CAD build for the part. Positions are in the model's coordinates, mm. A direction names the side the tool comes from. Give positions to 0.01 mm unless a question says otherwise; leave off trailing zeros. Write each loop counter-clockwise with the first axis right and the second up, starting at its lowest first coordinate (ties: lowest second). Pieces come first, ordered by that corner, then holes. Notation, with made-up numbers: (18, 62.5) - (27, 62.5) arc R15 ccw to (27, 73.5) - close; hole circle Ø2 at (75, 84). An arc over 180 degrees is marked (long way). Write item = value, one per line. Start each with the question number.
Autodesk Inventor part; units mm, degrees
ref_plane "YZ Plane" through (0, 0, 0) normal (1, 0, 0) x (0, 1, 0)
ref_plane "XZ Plane" through (0, 0, 0) normal (0, 1, 0) x (-1, 0, 0)
ref_plane "XY Plane" through (0, 0, 0) normal (0, 0, 1) x (1, 0, 0)
sketch "Sketch9" plane through (0, 0, 0) normal (0, 1, 0) x (-1, 0, 0)
  circle A0 centre (0, 0) radius 32
  circle A1 centre (0, 0) radius 47
  circle A2 centre (0, 0) radius 26.5
  dimension "d54" = 64
  dimension "d55" = 94
  dimension "d56" = 53
extrude "Extrusion8" add sketch "Sketch9" against normal blind 4 contours A0
extrude "Extrusion9" add sketch "Sketch9" against normal blind 10 contours A1
sketch "Sketch10" plane through (0, 0, 0) normal (0, 1, 0) x (1, 0, 0)
  circle A0 centre (0, 0) radius 40
  point P0 (-40, 0)
  point P1 (-30.6418, -25.7115)
  point P2 (-6.9459, -39.3923)
  point P3 (20, -34.641)
  point P4 (37.5877, -13.6808)
  point P5 (37.5877, 13.6808)
  point P6 (20, 34.641)
  point P7 (-6.9459, 39.3923)
  point P8 (-30.6418, 25.7115)
  dimension "d61" = 80
  dimension "d64" = 360
hole "Hole1" at (-40, 0, 0) at (-30.6418, 0, 25.7115) at (-6.9459, 0, 39.3923) at (20, 0, 34.641) at (37.5877, 0, 13.6808) at (37.5877, 0, -13.6808) at (20, 0, -34.641) at (-6.9459, 0, -39.3923) at (-30.6418, 0, -25.7115) direction (0, -1, 0) diameter 8 depth 5
hole "Hole2" at (-30.6418, 0, -25.7115) at (-6.9459, 0, -39.3923) at (20, 0, -34.641) at (37.5877, 0, -13.6808) at (37.5877, 0, 13.6808) at (-40, 0, 0) at (20, 0, 34.641) at (-6.9459, 0, 39.3923) at (-30.6418, 0, 25.7115) direction (0, -1, 0) diameter 4 depth 10
properties part number "GFK_Ring_oben" material "Default New Material"
1. Cut at B-B (z = 0). Give the cut face in (x, y).
2. Tool access for faces 1 (the cylindrical face through (35.6, -7.5, -13.9)), 2 (the cylindrical face through (-43.966, -2.535, -0.521)): list every direction of +Z, -Z, +X, -X, +Y, -Y with a clear straight run to the whole face (end or side of a thin tool).
3. Cut at D-D (z = -19.5). Give the cut face in (x, y), then the cut area to 3 significant figures.
4. Cut at C-C (y = -6.5). Count the separate pieces of the cut face and the enclosed holes in it, then the cut area to 3 significant figures.
5. Wall check: line 1 along Z through (x, y) = (-34, -4); line 2 along Z through (x, y) = (-10.5, -3); line 3 along Z through (x, y) = (20, -2.25). Give the ranges that are in metal, low to high.
6. Cut at A-A (x = 0). Give the cut face in (y, z).
7. Pin check, flat tips, straight feed: pin 1 Ø5 at (x, y) = (-15.5, -5.5) entering from -Z; pin 2 Ø2.5 at (x, z) = (37.59, -13.68) entering from -Y; pin 3 Ø6 at (y, z) = (-1, 8) entering from +X; pin 4 Ø5 at (x, y) = (2, -8.5) entering from +Z. Stop position of each tip, or through.
8. Mould opens along Z. For faces 3 (the flat face through (12, -4, 24)), 4 (the flat face through (-20, 0, -20)), 5 (the cylindrical face through (-44.83, -4.93, 14.12)) say: +Z half, -Z half, draft (parallel to the pull), parting line (faces both ways), or undercut.
Output:
q1.outline = (-47, -10) - (-42, -10) - (-42, -5) - (-44, -5) - (-44, 0) - (-47, 0) - close; (-38, -10) - (-32, -10) - (-32, -4) - (-26.5, -4) - (-26.5, 0) - (-36, 0) - (-36, -5) - (-38, -5) - close; (26.5, -4) - (32, -4) - (32, -10) - (47, -10) - (47, 0) - (26.5, 0) - close
q2.face_1 = +Y, -Y
q2.face_2 = +Y
q3.outline = (-42.76, -10) - (-25.37, -10) - (-25.37, -4) - (-17.94, -4) - (-17.94, 0) - (-42.76, 0) - close; (17.94, -4) - (25.37, -4) - (25.37, -10) - (42.76, -10) - (42.76, 0) - (17.94, 0) - close
q3.area = 407 mm2
q4.separate_pieces = 1
q4.enclosed_holes = 10
q4.area = 3,610 mm2
q5.line_1 = -32.45 to -27.88, -23.54 to 23.54, 27.88 to 32.45
q5.line_2 = -45.81 to -41.23, -37.56 to -24.33, 24.33 to 37.56, 41.23 to 45.81
q5.line_3 = -42.53 to -38.64, -30.64 to -17.39, 17.39 to 30.64, 38.64 to 42.53
q6.outline = (-10, -47) - (0, -47) - (0, -26.5) - (-4, -26.5) - (-4, -32) - (-10, -32) - close; (-10, 32) - (-4, 32) - (-4, 26.5) - (0, 26.5) - (0, 47) - (-10, 47) - close
q7.pin_1 = -45.17
q7.pin_2 = through
q7.pin_3 = 46.73
q7.pin_4 = 47
q8.face_3 = undercut
q8.face_4 = draft
q8.face_5 = parting line
